Here's how the part is built. I have some questions about the finished solid (model axes, mm). A direction names the side the tool comes from. Round coordinates to 2 decimals unless told otherwise and drop trailing zeros. Write each loop counter-clockwise with the first axis right and the second up, starting at its lowest first coordinate (ties: lowest second). Pieces come first, ordered by that corner, then holes. Notation, with made-up numbers: (81.25, -38) - (113.25, -38) arc R18 cw to (113.25, -14) - close; hole circle Ø5 at (37, 53.25). An arc over 180 degrees is marked (long way). Write item = value, one per line. Start each with the question number.
Item 1: Which directions (+Z, -Z, +X, -X, +Y, -Y) give clear straight access to the entire face, cutting with the end or side of a thin tool? Please do faces 4 (the face through (8.103, 97.874, 1.799)), 5 (the face through (9.7, 104, 0)), 6 (the face through (6.2, 88, -0.1)).
Item 2: Thinking about a two-plate mould opening in X: for faces 1 (the face through (0, 89, 0)), 2 (the face through (-1.802, 44.616, -5.723)), 3 (the face through (6, 107, -6)), which applies, pulls with the +X half, pulls with the -X half, needs draft (parallel to the pull), parting line crosses it, or undercut?
Item 3: If I drill on line 1 along X through (y, z) = (93.75, 0); line 2 along Z through (x, y) = (0.5, 79.5); line 3 along Y through (x, z) = (5.75, 4.5), over which ranges is the centre line in solid material (lowest first)? Write a range as [from, to].
Item 4: If we section it at C-C (y = 69): Please give me the cut outline in (x, z).
Item 5: If we section it at D-D (x = 5): Please give me the cut outline in (y, z), and give its area (3 significant figures).
Item 6: For P1, Ø1.5, axis at y = 45.5, z = 1, coming from the -X side; P2, Ø1.5, axis at y = 51, z = -2.5, coming from the -X side; P3, Ø1, axis at y = 57, z = 1.5, coming from the -X side, each with a flat end and sliding along its axis, tell me the tip position at first contact or that it passes through.
Item 7: If we section it at A-A (x = 0): Please give me the cut outline in (y, z), and give its area (3 significant figures).
Item 8: If we section it at B-B (z = 0): Please give me the cut outline in (x, y), and give its area (3 significant figures).
```python
from build123d import *

# Parameters (mm, degrees)
SKETCH_3_W          = 19.4
SKETCH_3_H          = 3
OUTPUT_KEY_DEPTH    = 5
D16_CLEARANCE_START = -18
SKETCH_4_R          = 8.3
D16_CLEARANCE_DEPTH = 18


with BuildPart() as part:
    # 草图1 → Stepped_output_tube (revolve)
    with BuildSketch(Plane.XY, mode=Mode.PRIVATE) as stepped_output_tube_sk:
        Polygon((0, 0), (6, 0), (6, 88), (9.5, 88), (9.5, 107), (8.3, 107), (8.3, 89), (0, 89), align=None)
    revolve(stepped_output_tube_sk.sketch.rotate(Axis((0, 0, 0), (0, 1, 0)), 90), axis=Axis((0, 0, 0), (0, 1, 0)))

    # 草图3 → Output_key (add)
    with BuildSketch(Plane.XY.offset(-2.5)):
        with Locations((0, 104.5)):
            Rectangle(SKETCH_3_W, SKETCH_3_H)
    extrude(amount=OUTPUT_KEY_DEPTH)

    # 草图4 → D16_clearance (cut)
    with BuildSketch(Plane(origin=(0, 107, 0), x_dir=(1, 0, 0), z_dir=(0, 1, 0)).offset(D16_CLEARANCE_START)):
        with Locations(Location((0, 0, 0), (0, 0, 90))):
            Circle(SKETCH_4_R)
    extrude(amount=D16_CLEARANCE_DEPTH, mode=Mode.SUBTRACT)


solid = part.part
```
Reply:
q1.face_4 = +Y
q1.face_5 = +Z, -Z, +X, +Y, -Y
q1.face_6 = -Y
q2.face_1 = undercut
q2.face_2 = parting line crosses it
q2.face_3 = needs draft
q3.line_1 = [-9.5, -8.3], [8.3, 9.5]
q3.line_2 = [-5.98, 5.98]
q3.line_3 = [88, 89]
q4.outline = circle Ø12 at (0, 0)
q5.outline = (0, -3.32) - (88, -3.32) - (88, -8.08) - (107, -8.08) - (107, -6.62) - (89, -6.62) - (89, 6.62) - (107, 6.62) - (107, 8.08) - (88, 8.08) - (88, 3.32) - (0, 3.32) - close
q5.area = 652 mm2
q6.P1 = -5.99
q6.P2 = -5.74
q6.P3 = -5.92
q7.outline = (0, -6) - (88, -6) - (88, -9.5) - (107, -9.5) - (107, -8.3) - (89, -8.3) - (89, 8.3) - (107, 8.3) - (107, 9.5) - (88, 9.5) - (88, 6) - (0, 6) - close
q7.area = 1,120 mm2
q8.outline = (-9.7, 103) - (-9.5, 103) - (-9.5, 88) - (-6, 88) - (-6, 0) - (6, 0) - (6, 88) - (9.5, 88) - (9.5, 103) - (9.7, 103) - (9.7, 106) - (9.5, 106) - (9.5, 107) - (8.3, 107) - (8.3, 89) - (-8.3, 89) - (-8.3, 107) - (-9.5, 107) - (-9.5, 106) - (-9.7, 106) - close
q8.area = 1,120 mm2
